Autodesk Inventor part; units mm, degrees
ref_plane "YZ Plane" through (0, 0, 0) normal (1, 0, 0) x (0, 1, 0)
ref_plane "XZ Plane" through (0, 0, 0) normal (0, 1, 0) x (-1, 0, 0)
ref_plane "XY Plane" through (0, 0, 0) normal (0, 0, 1) x (1, 0, 0)
sketch "Esboço1" plane through (0, 0, 0) normal (0, 0, 1) x (1, 0, 0)
  line L0 (30.4895, -39) -> (-329.5105, -39)
  line L1 (-329.5105, -39) -> (-329.5105, 6)
  line L2 (-329.5105, 6) -> (30.4895, 6)
  line L3 (30.4895, 6) -> (30.4895, -39)
  point P0 (0, 0)
  point P1 (-329.5105, 0)
  dimension "d0" = 45
extrude "Extrusão1" add sketch "Esboço1" along normal blind 9.52
sketch "Esboço2" plane through (0, 0, 9.52) normal (0, 0, 1) x (1, 0, 0)
  circle A0 centre (24.4895, -32.5) radius 2.067
  circle A1 centre (24.4895, -6.5) radius 2.067
  circle A2 centre (-3.5105, -6.5) radius 2.067
  circle A3 centre (-3.5105, -32.5) radius 2.067
  circle A4 centre (-323.5105, -32.5) radius 2.067
  circle A5 centre (-295.5105, -32.5) radius 2.067
  circle A6 centre (-295.5105, -6.5) radius 2.067
  circle A7 centre (-323.5105, -6.5) radius 2.067
  point P0 (0, 0)
hole "Furo1" at (24.4895, -32.5, 9.52) at (-3.5105, -32.5, 9.52) at (-3.5105, -6.5, 9.52) at (24.4895, -6.5, 9.52) at (-323.5105, -32.5, 9.52) at (-295.5105, -32.5, 9.52) at (-295.5105, -6.5, 9.52) at (-323.5105, -6.5, 9.52) direction (0, 0, -1) diameter 5.5 end through all counterbore diameter 7 counterbore depth 4
sketch "Esboço3" plane through (30.4895, -39, 0) normal (1, 0, 0) x (0, 0, -1)
  line L0 (0, 45) -> (-9.52, 45)
  line L1 (-9.52, 45) -> (-4.52, 42.1132)
  line L2 (-9.52, 45) -> (-3.7465, 45) construction
  line L3 (-4.52, 42.1132) -> (-4.52, 45)
  point P0 (0, 39)
  dimension "d10" = 30
  dimension "d13" = 5
extrude "Extrusão2" cut sketch "Esboço3" against normal through all
properties part number "SuportePincas"
Here's how the part is built. I have some questions about the finished solid (model axes, mm). A direction names the side the tool comes from. Coordinates: 2 decimals unless noted, no trailing zeros. Order: outer loops, then holes, each group sorted by start corner. A loop starts at its lowest first (then second) coordinate and runs counter-clockwise, first axis right, second up. Notation, with made-up numbers: (50, 12) -> (78, 12) arc R23 ccw to (78, 37) -> close; hole circle Ø2 at (18, 71.5). An arc over 180 degrees is marked (long way). Return JSON: item names as keys, results as strings.
1) On a 3-axis mill with a long thin cutter (end or side, diameter ignored), from which of +Z, -Z, +X, -X, +Y, -Y can I reach the whole of each face in a straight line? I mean faces 1 (the flat face through (-294, -4, 5.52)), 2 (the cylindrical face through (21.763, -6.142, 2.721)). Say none if no direction works.
Conclusion:
{"face 1": "+Z", "face 2": "+Z, -Z"}
2) I'm going to push flat-ended pins straight in: P1, Ø4, axis at x = -3.51, y = -32.5, coming from the -Z side; P2, Ø6.5, axis at x = 24.49, y = -32.5, coming from the +Z side. Where does each tip first touch, or does it pass through?
Conclusion:
{"P1": "passes through", "P2": "stops at z = 5.52"}
3) If I drill on probe 1 along X at (y, z) = (-6.5, 4.4); probe 2 along Y at (x, z) = (-83, 8.75); probe 3 along X at (y, z) = (-9.5, 6.25), over which ranges is the centre line in solid material (lowest first)?
Conclusion:
{"probe 1": "x = -329.51 to -326.26, -320.76 to -298.26, -292.76 to -6.26, -0.76 to 21.74, 27.24 to 30.49", "probe 2": "y = -39 to 5.56", "probe 3": "x = -329.51 to -325.31, -321.71 to -297.31, -293.71 to -5.31, -1.71 to 22.69, 26.29 to 30.49"}
4) If we section it at A-A on x = -167.5: List the corners of the cut face in (y, z) for me.
Conclusion:
{"outline": "(-39, 0) -> (6, 0) -> (6, 4.52) -> (3.11, 4.52) -> (6, 9.52) -> (-39, 9.52) -> close"}
5) Thinking about a two-plate mould opening in Y: for faces 3 (the cylindrical face through (-297.83, -7.98, 2.72)), 4 (the flat face through (-147, -39, 5)), 5 (the flat face through (-152, -16, 9.52)), 6 (the flat face through (26, -4, 5.52)), which applies, +Y half, -Y half, draft (parallel to the pull), parting line (faces both ways), or undercut?
Conclusion:
{"face 3": "undercut", "face 4": "-Y half", "face 5": "draft", "face 6": "undercut"}
